from build123d import *

# Parameters (mm, degrees)
CROQUIS1_W              = 50.8
CROQUIS1_H              = 86
SALIENTE_EXTRUIR1_DEPTH = 6.35
CROQUIS2_R              = 4
CROQUIS2_R_2            = 2.6
CORTAR_EXTRUIR1_DEPTH   = 6.35
CROQUIS3_R              = 1.785
CORTAR_EXTRUIR2_DEPTH   = 7.35


with BuildPart() as part:
    # Croquis1 → Saliente-Extruir1 (new body)
    with BuildSketch(Plane.XY):
        with Locations((25.4, 43)):
            Rectangle(CROQUIS1_W, CROQUIS1_H)
    extrude(amount=SALIENTE_EXTRUIR1_DEPTH)

    # Croquis2 → Cortar-Extruir1 (cut)
    with BuildSketch(Plane.XY.offset(6.35)):
        with Locations((25.4, 43)):
            Circle(CROQUIS2_R)
        with Locations((25.4, 61.25)):
            Circle(CROQUIS2_R_2)
        with Locations((25.4, 24.75)):
            Circle(CROQUIS2_R_2)
    extrude(amount=-CORTAR_EXTRUIR1_DEPTH, mode=Mode.SUBTRACT)

    # Croquis3 → Cortar-Extruir2 (cut, through all)
    with BuildSketch(Plane.XY.offset(6.35)):
        with Locations((25.4, 81)):
            Circle(CROQUIS3_R)
        with Locations((11.4, 77)):
            Circle(CROQUIS3_R)
        with Locations((39.4, 77)):
            Circle(CROQUIS3_R)
        with Locations((39.4, 9)):
            Circle(CROQUIS3_R)
        with Locations((11.4, 9)):
            Circle(CROQUIS3_R)
        with Locations((25.4, 5)):
            Circle(CROQUIS3_R)
    extrude(amount=-CORTAR_EXTRUIR2_DEPTH, mode=Mode.SUBTRACT)


solid = part.part
The listing builds one solid part. Answer for the finished solid, in the listing's coordinates (mm). Round coordinates to 2 decimals unless told otherwise and drop trailing zeros. Order: outer loops, then holes, each group sorted by start corner. A loop starts at its lowest first (then second) coordinate and runs counter-clockwise, first axis right, second up. Notation, with made-up numbers: M 69.25,-31 L 114.25,-31 A11 cw 114.25,-20 Z; hole C 71,82.5 d5. An arc over 180 degrees is marked long. Answer in a Markdown table with one row per item. Add a question column.
1) The part is cut by section C-C on x = 25.4. Determine the outline of the cut face in (y, z) (3 decimals), plus the area to 3 significant figures.
2) Determine the mould class of faces 1 (the face through (25, 0, 3)), 2 (the face through (29.215, 44.201, 3.219)), 3 (the face through (13.05, 8.32, 3.22)), 4 (the face through (0, 42, 3)) for opening direction X: pulls with the +X half, pulls with the -X half, needs draft (parallel to the pull), parting line crosses it, or undercut.
3) The part is cut by section D-D on y = 24.75. Determine the outline of the cut face in (x, z).
4) The part is cut by section B-B on z = 3. Count the separate pieces of the cut face and the enclosed holes in it, plus the area to 3 significant figures.
5) The part is cut by section A-A on y = 9. Determine the outline of the cut face in (x, z) (3 decimals).
6) Flat-ended cylindrical pins translate along their axes: pin 1 Ø3 at (x, y) = (39.4, 77) entering from -Z (3 decimals); pin 2 Ø7 at (x, y) = (25.4, 61.25) entering from -Z. Find the tip coordinate at first contact, or state that the pin passes through.
7) Consider line 1 along Y through (x, z) = (11.4, 2.75) (3 decimals); line 2 along Y through (x, z) = (25.4, 4) (3 decimals); line 3 along X through (y, z) = (76.5, 1). Determine where each line is inside the solid, lowest interval first. Write a range as from..to.
Findings below:
| question | item | result |
|---|---|---|
| 1 | outline | M 0,0 L 3.215,0 L 3.215,6.35 L 0,6.35 Z; M 6.785,0 L 22.15,0 L 22.15,6.35 L 6.785,6.35 Z; M 27.35,0 L 39,0 L 39,6.35 L 27.35,6.35 Z; M 47,0 L 58.65,0 L 58.65,6.35 L 47,6.35 Z; M 63.85,0 L 79.215,0 L 79.215,6.35 L 63.85,6.35 Z; M 82.785,0 L 86,0 L 86,6.35 L 82.785,6.35 Z |
| 1 | area | 384 mm² |
| 2 | face 1 | needs draft |
| 2 | face 2 | undercut |
| 2 | face 3 | undercut |
| 2 | face 4 | pulls with the -X half |
| 3 | outline | M 0,0 L 22.8,0 L 22.8,6.35 L 0,6.35 Z; M 28,0 L 50.8,0 L 50.8,6.35 L 28,6.35 Z |
| 4 | separate pieces | 1 |
| 4 | enclosed holes | 9 |
| 4 | area | 4,220 mm² |
| 5 | outline | M 0,0 L 9.615,0 L 9.615,6.35 L 0,6.35 Z; M 13.185,0 L 37.615,0 L 37.615,6.35 L 13.185,6.35 Z; M 41.185,0 L 50.8,0 L 50.8,6.35 L 41.185,6.35 Z |
| 6 | pin 1 | passes through |
| 6 | pin 2 | stops at z = 0 |
| 7 | line 1 | y = 0..7.215, 10.785..75.215, 78.785..86 |
| 7 | line 2 | y = 0..3.215, 6.785..22.15, 27.35..39, 47..58.65, 63.85..79.215, 82.785..86 |
| 7 | line 3 | x = 0..9.69, 13.11..37.69, 41.11..50.8 |
